CAD build for the part. Positions are in the model's coordinates, mm. Face numbers are marked on the shaded views. A direction names the side the tool comes from. Give positions to 0.01 mm unless a question says otherwise; leave off trailing zeros. Order: outer loops, then holes, each group sorted by start corner. A loop starts at its lowest first (then second) coordinate and runs counter-clockwise, first axis right, second up. Notation, with made-up numbers: (-38, 10.5) -> (18, 10.5) arc R22 cw to (18, 47.5) -> close; hole circle Ø4 at (65.25, 57.5). An arc over 180 degrees is marked (long way). Use one line per item in the form item = value. Start each with the question number.
1) Tool access for the marked faces 4, 5 and 6: list every direction of +Z, -Z, +X, -X, +Y, -Y with a clear straight run to the whole face (end or side of a thin tool).
2) Cut at C-C, the plane y = 5. Give the cut face in (x, z).
3) Cut at A-A, the plane y = 24.5. Give the cut face in (x, z).
4) Drop flat-ended pins along their axis: P1, Ø4.5, axis at x = 47, z = -5, coming from the +Y side; P2, Ø4.5, axis at x = -48.5, y = 37, coming from the +Z side; P3, Ø2, axis at x = 0, y = 6.5, coming from the +Z side. Give the stop position or say it passes through.
5) Mould opens along X. For the marked faces 1, 2 and 3 say: pulls with the +X half, pulls with the -X half, needs draft (parallel to the pull), parting line crosses it, or undercut.
6) Cut at D-D, the plane x = 0. Give the cut face in (y, z), and give its area (3 significant figures).
7) Cut at B-B, the plane z = 42. Give the cut face in (x, y).
8) Probe line 1 (X direction, y = 14, z = 1); line 2 (Y direction, x = 30, z = 35); line 3 (X direction, y = 7, z = 24). List the from-to ranges inside material, lowest first.
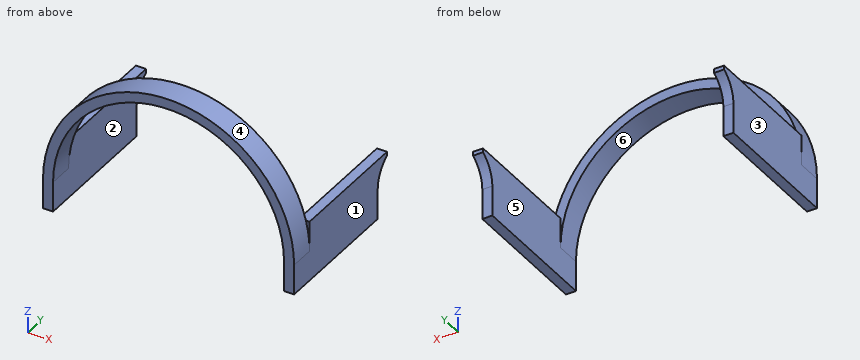
from build123d import *

# Parameters (mm, degrees)
EXTRUDE_1_DEPTH     = 10
SKETCH_2_W          = 4
SKETCH_2_H          = 24
EXTRUDE_2_DEPTH     = 50
CUT_EXTRUDE_3_DEPTH = 127.885775404


with BuildPart() as part:
    # 草图1 → 凸台-拉伸1 (new body)
    with BuildSketch(Plane(origin=(0, 0, 0), x_dir=(1, 0, 0), z_dir=(0, 1, 0))):
        with BuildLine():
            Line((-50, 12), (-46, 12))
            Line((-46, 12), (-46, 0))
            ThreePointArc((-46, 0), (0, -46), (46, 0))
            Line((46, 0), (46, 12))
            Line((46, 12), (50, 12))
            Line((50, 12), (50, 0))
            ThreePointArc((50, 0), (0, -50), (-50, 0))
            Line((-50, 0), (-50, 12))
        make_face()
    extrude(amount=EXTRUDE_1_DEPTH)

    # 草图2 → 凸台-拉伸2 (add)
    with BuildSketch(Plane(origin=(0, 10, 0), x_dir=(1, 0, 0), z_dir=(0, 1, 0))):
        with Locations((-48, 0)):
            Rectangle(SKETCH_2_W, SKETCH_2_H)
        with Locations((48, 0)):
            Rectangle(SKETCH_2_W, SKETCH_2_H)
    extrude(amount=EXTRUDE_2_DEPTH)

    # 草图3 → 切除-拉伸3 (cut, through all)
    with BuildSketch(Plane(origin=(50, 0, 0), x_dir=(0, 0, -1), z_dir=(1, 0, 0))):
        with BuildLine():
            Line((0, 54), (12, 54))
            Line((12, 54), (12, 66))
            ThreePointArc((12, 66), (-8.485281374, 74.485281374), (0, 54))
        make_face()
    extrude(amount=-CUT_EXTRUDE_3_DEPTH, mode=Mode.SUBTRACT)


solid = part.part
Result:
q1.face_4 = +Z, -Y
q1.face_5 = -Z, +Y
q1.face_6 = -Z, +Y, -Y
q2.outline = (-50, -12) -> (-46, -12) -> (-46, 0) arc R46 cw to (46, 0) -> (46, -12) -> (50, -12) -> (50, 0) arc R50 ccw to (-50, 0) -> close
q3.outline = (-50, -12) -> (-46, -12) -> (-46, 12) -> (-50, 12) -> close; (46, -12) -> (50, -12) -> (50, 12) -> (46, 12) -> close
q4.P1 = 54
q4.P2 = 12
q4.P3 = 50
q5.face_1 = pulls with the +X half
q5.face_2 = undercut
q5.face_3 = pulls with the -X half
q6.outline = (0, 46) -> (10, 46) -> (10, 50) -> (0, 50) -> close
q6.area = 40.0 mm²
q7.outline = (-27.13, 0) -> (-18.76, 0) -> (-18.76, 10) -> (-27.13, 10) -> close; (18.76, 0) -> (27.13, 0) -> (27.13, 10) -> (18.76, 10) -> close
q8.line_1 = -50 to -46, 46 to 50
q8.line_2 = 0 to 10
q8.line_3 = -43.86 to -39.24, 39.24 to 43.86
